```python
from build123d import *

# Parameters (mm, degrees)
SKETCH1_W           = 20.3
SKETCH1_H           = 40.5
BOSS_EXTRUDE1_DEPTH = 36.5
SKETCH4_W           = 20.3
SKETCH4_H           = 2.3
BOSS_EXTRUDE4_DEPTH = 6.8
SKETCH5_R           = 2.3
CUT_EXTRUDE1_DEPTH  = 2.3
BOSS_EXTRUDE5_DEPTH = 2.5
SKETCH10_R          = 6.45
BOSS_EXTRUDE6_DEPTH = 2
SKETCH11_R          = 5.65
BOSS_EXTRUDE7_DEPTH = 0.5
SKETCH12_R          = 3
BOSS_EXTRUDE8_DEPTH = 4
SKETCH13_R          = 1.15
CUT_EXTRUDE2_DEPTH  = 4
SKETCH14_W          = 17.3
SKETCH14_H          = 12
CUT_EXTRUDE3_DEPTH  = 0.5


with BuildPart() as part:
    # Sketch1 → Boss-Extrude1 (new body)
    with BuildSketch(Plane(origin=(0, 0, 0), x_dir=(1, 0, 0), z_dir=(0, 1, 0))):
        Rectangle(SKETCH1_W, SKETCH1_H)
    extrude(amount=BOSS_EXTRUDE1_DEPTH)

    # Sketch4 → Boss-Extrude4 (add)
    with BuildSketch(Plane.XY.offset(20.25)):
        with Locations((0, 29.75)):
            Rectangle(SKETCH4_W, SKETCH4_H)
    boss_extrude4 = extrude(amount=BOSS_EXTRUDE4_DEPTH)

    # Sketch5 → Cut-Extrude1 (cut)
    with BuildSketch(Plane(origin=(0, 30.9, 0), x_dir=(1, 0, 0), z_dir=(0, 1, 0))):
        with Locations((5.75, -24.85)):
            Circle(SKETCH5_R)
        with Locations((-5.75, -24.85)):
            Circle(SKETCH5_R)
    cut_extrude1 = extrude(amount=-CUT_EXTRUDE1_DEPTH, mode=Mode.SUBTRACT)

    # Mirror2: Boss-Extrude4, Cut-Extrude1 across plane
    add(boss_extrude4.mirror(Plane.XY))
    add(cut_extrude1.mirror(Plane.XY), mode=Mode.SUBTRACT)

    # Sketch7 → Boss-Extrude5 (add)
    with BuildSketch(Plane(origin=(0, 36.5, 0), x_dir=(1, 0, 0), z_dir=(0, 1, 0))):
        with BuildLine():
            Line((-9.65, 14.25), (-9.65, -7.05))
            ThreePointArc((-9.65, -7.05), (0, -20.25), (9.65, -7.05))
            Line((9.65, -7.05), (9.65, 14.25))
            Line((9.65, 14.25), (-9.65, 14.25))
        make_face()
    extrude(amount=BOSS_EXTRUDE5_DEPTH)

    # Sketch10 → Boss-Extrude6 (add)
    with BuildSketch(Plane(origin=(0, 39, 0), x_dir=(1, 0, 0), z_dir=(0, 1, 0))):
        with Locations((0, -11.25)):
            Circle(SKETCH10_R)
    extrude(amount=BOSS_EXTRUDE6_DEPTH)

    # Sketch11 → Boss-Extrude7 (add)
    with BuildSketch(Plane(origin=(0, 41, 0), x_dir=(1, 0, 0), z_dir=(0, 1, 0))):
        with Locations((0, -11.25)):
            Circle(SKETCH11_R)
    extrude(amount=BOSS_EXTRUDE7_DEPTH)

    # Sketch12 → Boss-Extrude8 (add)
    with BuildSketch(Plane(origin=(0, 41.5, 0), x_dir=(1, 0, 0), z_dir=(0, 1, 0))):
        with Locations((0, -11.25)):
            Circle(SKETCH12_R)
    extrude(amount=BOSS_EXTRUDE8_DEPTH)

    # Sketch13 → Cut-Extrude2 (cut)
    with BuildSketch(Plane(origin=(0, 45.5, 0), x_dir=(1, 0, 0), z_dir=(0, 1, 0))):
        with Locations((0, -11.25)):
            Circle(SKETCH13_R)
    extrude(amount=-CUT_EXTRUDE2_DEPTH, mode=Mode.SUBTRACT)

    # Sketch14 → Cut-Extrude3 (cut)
    with BuildSketch(Plane(origin=(0, 39, 0), x_dir=(1, 0, 0), z_dir=(0, 1, 0))):
        with Locations((0, 7.25)):
            Rectangle(SKETCH14_W, SKETCH14_H)
    extrude(amount=-CUT_EXTRUDE3_DEPTH, mode=Mode.SUBTRACT)


solid = part.part
```
Part model, mm, in its own coordinate system. A direction names the side the tool comes from. Give positions to 0.01 mm unless a question says otherwise; leave off trailing zeros. Write each loop counter-clockwise with the first axis right and the second up, starting at its lowest first coordinate (ties: lowest second). Pieces come first, ordered by that corner, then holes. Notation, with made-up numbers: (-7, 61) -> (22, 61) arc R13 ccw to (22, 79) -> close; hole circle Ø4 at (65.25, 8). An arc over 180 degrees is marked (long way). Put each result on its own line as item: value. Start each with the question number.
Item 1: Pull direction Z, two halves, no side cores. Call faces 4 (the face through (10.15, 18, 0)), 5 (the face through (5.84, 29.77, -22.55)), 6 (the face through (0, 14, 20.25)): pulls with the +Z half, pulls with the -Z half, needs draft (parallel to the pull), parting line crosses it, or undercut.
Item 2: Which spindle directions (+Z, -Z, +X, -X, +Y, -Y) get a long thin tool onto all of the face, cutting with end or side? Do faces 1 (the face through (9.65, 38, -3)), 2 (the face through (0, 30.9, -23)), 3 (the face through (-0.266, 37.732, 20.246)). Say none if no direction does.
Item 3: Cut at A-A (z = -24.85). List the corners of the cut face in (x, y).
Item 4: Pin check, flat tips, straight feed: pin 1 Ø1 at (x, z) = (-1, 18) entering from -Y; pin 2 Ø6 at (x, z) = (-5.75, -24.85) entering from +Y; pin 3 Ø0.7 at (x, z) = (0, 10.5) entering from +Y; pin 4 Ø10 at (x, y) = (-5, 12.5) entering from +Z. Stop position of each tip, or through.
Item 5: Cut at C-C (z = -8). List the corners of the cut face in (x, y), then the cut area to 3 significant figures.
Item 6: Cut at D-D (y = 8). List the corners of the cut face in (x, z), then the cut area to 3 significant figures.
Item 7: Wall check: L1, parallel to X at y = 29.35, z = -24.85; L2, parallel to X at y = 43.5, z = 11.25; L3, parallel to Z at x = 0, y = 42.8. Give the ranges that are in metal, low to high. Write a range as [from, to].
Answer list:
1. face 4: needs draft
1. face 5: undercut
1. face 6: pulls with the +Z half
2. face 1: -Z, +X, +Y
2. face 2: -Z, +X, -X, +Y
2. face 3: +Y
3. outline: (-10.15, 28.6) -> (-8.05, 28.6) -> (-8.05, 30.9) -> (-10.15, 30.9) -> close; (-3.45, 28.6) -> (3.45, 28.6) -> (3.45, 30.9) -> (-3.45, 30.9) -> close; (8.05, 28.6) -> (10.15, 28.6) -> (10.15, 30.9) -> (8.05, 30.9) -> close
4. pin 1: stops at y = 0
4. pin 2: stops at y = 30.9
4. pin 3: stops at y = 41.5
4. pin 4: stops at z = 20.25
5. outline: (-10.15, 0) -> (10.15, 0) -> (10.15, 36.5) -> (9.65, 36.5) -> (9.65, 39) -> (8.65, 39) -> (8.65, 38.5) -> (-8.65, 38.5) -> (-8.65, 39) -> (-9.65, 39) -> (-9.65, 36.5) -> (-10.15, 36.5) -> close
5. area: 781 mm2
6. outline: (-10.15, -20.25) -> (10.15, -20.25) -> (10.15, 20.25) -> (-10.15, 20.25) -> close
6. area: 822 mm2
7. L1: x = [-10.15, -8.05], [-3.45, 3.45], [8.05, 10.15]
7. L2: x = [-3, -1.15], [1.15, 3]
7. L3: z = [8.25, 10.1], [12.4, 14.25]
